Source: CAD feature listing. Evaluate the final solid. Frame: model axes, mm. Give positions to 0.01 mm unless a question says otherwise; leave off trailing zeros. Loops run counter-clockwise (first coordinate to the right, second up) from the corner with the lowest first, then second, coordinate; pieces in that order, holes last.
from build123d import *

# Parameters (mm, degrees)
SKETCH1_R           = 10
BOSS_EXTRUDE1_DEPTH = 2.5
SKETCH2_R           = 7.5
BOSS_EXTRUDE2_DEPTH = 0.5


with BuildPart() as part:
    # Sketch1 → Boss-Extrude1 (new body)
    with BuildSketch(Plane(origin=(0, 0, 0), x_dir=(1, 0, 0), z_dir=(0, 1, 0))):
        with Locations(Location((0, 0, 0), (0, 0, 270))):
            Circle(SKETCH1_R)
    extrude(amount=BOSS_EXTRUDE1_DEPTH)

    # Sketch2 → Boss-Extrude2 (add)
    with BuildSketch(Plane(origin=(0, 2.5, 0), x_dir=(1, 0, 0), z_dir=(0, 1, 0))):
        with Locations(Location((0, 0, 0), (0, 0, 270))):
            Circle(SKETCH2_R)
    extrude(amount=BOSS_EXTRUDE2_DEPTH)

    # Sketch4 → CSK for M3 Hex Socket Countersunk Head Screw1 (revolve, cut)
    with BuildSketch(Plane(origin=(0, 0, 0), x_dir=(0, 0, -1), z_dir=(1, 0, 0))):
        Polygon((0, 0), (0, 3), (1.8, 3), (1.8, 1.67), (3.47, 0), align=None)
    revolve(axis=Axis((0, -6.35, 0), (0, 1, 0)), mode=Mode.SUBTRACT)


solid = part.part
1) Pull-direction query (X, two-part tool) for faces 1 (the cylindrical face through (-0.541, 2.326, -1.717)), 2 (the flat face through (7, 2.5, 4)), 3 (the cylindrical face through (0.33, 2.746, -7.493)); classes: released by +X, released by -X, zero draft, split by the parting line, or undercut.
Checks:
face 1: undercut
face 2: zero draft
face 3: split by the parting line
2) Cut plane A-A (x = 0). Return loops of the section in (y, z), and give its area (3 significant figures).
Checks:
outline: (0, -10) - (2.5, -10) - (2.5, -7.5) - (3, -7.5) - (3, -1.8) - (1.67, -1.8) - (0, -3.47) - close; (0, 3.47) - (1.67, 1.8) - (3, 1.8) - (3, 7.5) - (2.5, 7.5) - (2.5, 10) - (0, 10) - close
area: 43.9 mm2
3) Cut plane D-D (x = -5). Return loops of the section in (y, z).
Checks:
outline: (0, -8.66) - (2.5, -8.66) - (2.5, -5.59) - (3, -5.59) - (3, 5.59) - (2.5, 5.59) - (2.5, 8.66) - (0, 8.66) - close
4) Contact query for flat-ended pins moving along their axis: P1, Ø1.5, axis at y = 0.5, z = 3, coming from the +X side; P2, Ø1, axis at x = -1.5, z = -1.5, coming from the -Y side; P3, Ø4.5, axis at x = 0, z = 0, coming from the +Y side; P4, Ø1.5, axis at y = 2.5, z = 2, coming from the -X side. Output: stop coordinate, or through.
Checks:
P1: stops at x = 9.74
P2: stops at y = 0.85
P3: stops at y = 3
P4: stops at x = -9.92
5) Cut plane B-B (z = 0). Return loops of the section in (x, y), and give its area (3 significant figures).
Checks:
outline: (-10, 0) - (-3.47, 0) - (-1.8, 1.67) - (-1.8, 3) - (-7.5, 3) - (-7.5, 2.5) - (-10, 2.5) - close; (1.8, 1.67) - (3.47, 0) - (10, 0) - (10, 2.5) - (7.5, 2.5) - (7.5, 3) - (1.8, 3) - close
area: 43.9 mm2
6) Cut plane C-C (z = 4.75). Return loops of the section in (x, y), and give its area (3 significant figures).
Checks:
outline: (-8.8, 0) - (8.8, 0) - (8.8, 2.5) - (5.8, 2.5) - (5.8, 3) - (-5.8, 3) - (-5.8, 2.5) - (-8.8, 2.5) - close
area: 49.8 mm2
7) Ray query, probe 1 along X at (y, z) = (2.25, 0); probe 2 along X at (y, z) = (2.6, 0); probe 3 along Z at (x, y) = (-0.25, 2.8). Return the intervals inside material, ascending.
Checks:
probe 1: x = -10 to -1.8, 1.8 to 10
probe 2: x = -7.5 to -1.8, 1.8 to 7.5
probe 3: z = -7.5 to -1.78, 1.78 to 7.5
